Verification items for the finished model (mm, model axes). A direction names the side the tool comes from. Give positions to 0.01 mm unless a question says otherwise; leave off trailing zeros. Answer as a JSON object with one key per item and string values.
```python
from build123d import *

# Parameters (mm, degrees)
SKETCH1_W            = 62.519999928
SKETCH1_H            = 66.675
BOSS_EXTRUDE1_DEPTH  = 2.929999982
SKETCH2_W            = 2.929999982
SKETCH2_H            = 33.3375
CUT_EXTRUDE1_DEPTH   = 3.929999982
BOSS_EXTRUDE2_DEPTH  = 2.93
FILLET1_R            = 0.2
SKETCH5_R            = 0.25
CUT_EXTRUDE2_DEPTH   = 3.93
FILLET2_R            = 0.5
FILLET1_OF_MIRROR1_R = 0.2
FILLET2_OF_MIRROR1_R = 0.5


with BuildPart() as part:
    # Sketch1 → Boss-Extrude1 (new body)
    with BuildSketch(Plane.XY):
        Rectangle(SKETCH1_W, SKETCH1_H)
    extrude(amount=BOSS_EXTRUDE1_DEPTH)

    # Sketch2 → Cut-Extrude1 (cut, through all)
    with BuildSketch(Plane.XY.offset(2.929999982)):
        with Locations((-26.864999991, -16.66875)):
            Rectangle(SKETCH2_W, SKETCH2_H)
    cut_extrude1 = extrude(amount=-CUT_EXTRUDE1_DEPTH, mode=Mode.SUBTRACT)

    # Sketch4 → Boss-Extrude2 (add)
    with BuildSketch(Plane.XY.offset(2.929999982)):
        Polygon((-27.330001982, -30.407500018), (-28.329999982, -30.407500018), (-28.329999982, -32.407498018), (-27.330001982, -31.407500018), align=None)
    boss_extrude2 = extrude(amount=-BOSS_EXTRUDE2_DEPTH)

    # Fillet1
    fillet1_edges = [part.edges().sort_by_distance(p)[0] for p in [
        (-27.330001982, -30.407500018, 1.464999982),
        (-28.329999982, -32.407498018, 1.464999982),
        (-27.330001982, -31.407500018, 1.464999982),
    ]]
    fillet(fillet1_edges, radius=FILLET1_R)

    # Sketch5 → Cut-Extrude2 (cut, through all)
    with BuildSketch(Plane.XY.offset(2.929999982)):
        with Locations((-28.329999982, 0)):
            Circle(SKETCH5_R)
    cut_extrude2 = extrude(amount=-CUT_EXTRUDE2_DEPTH, mode=Mode.SUBTRACT)

    # Fillet2
    fillet2_edges = [part.edges().sort_by_distance(p)[0] for p in [
        (-28.079999982, 0, 1.464999991),
        (-28.329999982, -0.25, 1.464999991),
    ]]
    fillet(fillet2_edges, radius=FILLET2_R)

    # Mirror1: Cut-Extrude1, Boss-Extrude2, Cut-Extrude2 across plane
    add(cut_extrude1.mirror(Plane(origin=(0, 0, 0), x_dir=(0, 0, 1), z_dir=(1, 0, 0))), mode=Mode.SUBTRACT)
    add(boss_extrude2.mirror(Plane(origin=(0, 0, 0), x_dir=(0, 0, 1), z_dir=(1, 0, 0))))
    add(cut_extrude2.mirror(Plane(origin=(0, 0, 0), x_dir=(0, 0, 1), z_dir=(1, 0, 0))), mode=Mode.SUBTRACT)

    # Fillet1 of Mirror1
    fillet1_of_mirror1_edges = [part.edges().sort_by_distance(p)[0] for p in [
        (27.330001982, -30.407500018, 1.464999982),
        (28.329999982, -32.407498018, 1.464999982),
        (27.330001982, -31.407500018, 1.464999982),
    ]]
    fillet(fillet1_of_mirror1_edges, radius=FILLET1_OF_MIRROR1_R)

    # Fillet2 of Mirror1
    fillet2_of_mirror1_edges = [part.edges().sort_by_distance(p)[0] for p in [
        (28.079999982, 0, 1.464999991),
        (28.329999982, -0.25, 1.464999991),
    ]]
    fillet(fillet2_of_mirror1_edges, radius=FILLET2_OF_MIRROR1_R)


solid = part.part
```
(1) Gauge pin test, flat end, axial feed: pin 1 Ø1.2 at (x, z) = (27, 2) entering from -Y. Record the tip position at first contact, or that the pin passes through.
Computed values:
{"pin 1": "stops at y = -31.68"}
(2) Access from +Z, -Z, +X, -X, +Y, -Y to the whole of each face (thin tool, end or side, straight path). Record for faces 4 (the flat face through (27, 0, 1)), 5 (the flat face through (-25.4, -17, 1)), 6 (the flat face through (30, -33.338, 1)).
Computed values:
{"face 4": "+Z, -Z", "face 5": "+Z, -Z, -Y", "face 6": "+Z, -Z, +X, -X, -Y"}
(3) Material ranges on line 1 along X through (y, z) = (-23.5, 1.6); line 2 along Y through (x, z) = (28, 0.85), recorded low to high. Write a range as [from, to].
Computed values:
{"line 1": "x = [-31.26, -28.33], [-25.4, 25.4], [28.33, 31.26]", "line 2": "y = [-32.08, -30.41], [0.06, 33.34]"}
(4) Release check for a two-part mould opening along Y. For faces 1 (the flat face through (0, 33.338, 1)), 2 (the flat face through (28.33, -16, 1)), 3 (the flat face through (25.4, -17, 1)) record: pulls with the +Y half, pulls with the -Y half, needs draft (parallel to the pull), parting line crosses it, or undercut.
Computed values:
{"face 1": "pulls with the +Y half", "face 2": "undercut", "face 3": "needs draft"}
